Could you check a few things on this model? Use its own coordinates, in mm. A direction names the side the tool comes from. Give positions to 0.01 mm unless a question says otherwise; leave off trailing zeros. Loops run counter-clockwise (first coordinate to the right, second up) from the corner with the lowest first, then second, coordinate; pieces in that order, holes last. Notation, with made-up numbers: (25, 37) - (68, 37) arc R25 ccw to (68, 63) - close; hole circle Ø3 at (-20, -14). An arc over 180 degrees is marked (long way). Use CSV: the item, a comma, the result in double quotes.
from build123d import *

# Parameters (mm, degrees)
SKETCH1_W       = 10
SKETCH1_H       = 16.5
MAIN_BODY_DEPTH = 12.2
M_BASE_DEPTH    = 4.95
SKETCH12_W      = 4.5
SKETCH12_H      = 1
MO_CUT_1_DEPTH  = 6
SKETCH13_W      = 1
SKETCH13_H      = 1
MO_PINS_DEPTH   = 5


with BuildPart() as part:
    # Sketch1 → Main_Body (new body)
    with BuildSketch(Plane(origin=(0, 0, 0), x_dir=(1, 0, 0), z_dir=(0, 1, 0))):
        with Locations((0, 8.25)):
            Rectangle(SKETCH1_W, SKETCH1_H)
    extrude(amount=MAIN_BODY_DEPTH)

    # Sketch11 → M_Base (add, symmetric)
    with BuildSketch(Plane(origin=(0, 0, 0), x_dir=(0, 0, -1), z_dir=(1, 0, 0))):
        Polygon((0.7, 12.2), (1.063619422, 17.4), (22.553619422, 17.4), (22.553619422, 10.8), (16.5, 10.8), (16.5, 12.2), align=None)
    extrude(amount=M_BASE_DEPTH, both=True)

    # Sketch12 → MO_Cut_1 (cut)
    with BuildSketch(Plane(origin=(0, 0, -22.553619422), x_dir=(-1, 0, 0), z_dir=(0, 0, -1))):
        with Locations((0, 16.9)):
            Rectangle(SKETCH12_W, SKETCH12_H)
        Polygon((-3.45, 15.1), (3.45, 15.1), (3.45, 13.6), (2.9, 13.6), (2.9, 11.9), (-2.9, 11.9), (-2.9, 13.6), (-3.45, 13.6), align=None)
    extrude(amount=-MO_CUT_1_DEPTH, mode=Mode.SUBTRACT)

    # Sketch13 → MO_Pins (add)
    with BuildSketch(Plane(origin=(0, 0, -16.553619422), x_dir=(-1, 0, 0), z_dir=(0, 0, -1))):
        with Locations((-1.25, 13.8)):
            Rectangle(SKETCH13_W, SKETCH13_H)
        with Locations((1.25, 13.8)):
            Rectangle(SKETCH13_W, SKETCH13_H)
    extrude(amount=MO_PINS_DEPTH)


solid = part.part
1) Suppose I cut it at A-A (z = -18.5). Please give me the cut outline in (x, y), plus the area to 3 significant figures.
Answer below:
outline,"(-4.95, 10.8) - (4.95, 10.8) - (4.95, 17.4) - (2.25, 17.4) - (2.25, 16.4) - (-2.25, 16.4) - (-2.25, 17.4) - (-4.95, 17.4) - close; (-1.75, 13.3) - (-0.75, 13.3) - (-0.75, 14.3) - (-1.75, 14.3) - close; (0.75, 13.3) - (1.75, 13.3) - (1.75, 14.3) - (0.75, 14.3) - close; hole (-3.45, 13.6) - (-2.9, 13.6) - (-2.9, 11.9) - (2.9, 11.9) - (2.9, 13.6) - (3.45, 13.6) - (3.45, 15.1) - (-3.45, 15.1) - close"
area,"42.6 mm2"
2) Suppose I cut it at D-D (x = 4.25). Please give me the cut outline in (y, z), plus the area to 3 significant figures.
Answer below:
outline,"(0, -16.5) - (10.8, -16.5) - (10.8, -22.55) - (17.4, -22.55) - (17.4, -1.06) - (12.2, -0.7) - (12.2, 0) - (0, 0) - close"
area,"322 mm2"
3) Suppose I cut it at C-C (y = 3). Please give me the cut outline in (x, z).
Answer below:
outline,"(-5, -16.5) - (5, -16.5) - (5, 0) - (-5, 0) - close"
4) We'd pull the mould along X, two halves only. Please class faces 1 (the flat face through (-3.45, 14, -20)), 2 (the flat face through (0, 17.4, -12)), 3 (the flat face through (5, 6, -8)): +X half, -X half, draft (parallel to the pull), parting line (faces both ways), or undercut.
Answer below:
face 1,"undercut"
face 2,"draft"
face 3,"+X half"
5) Suppose I cut it at B-B (x = -0.5). Please give me the cut outline in (y, z).
Answer below:
outline,"(0, -16.5) - (10.8, -16.5) - (10.8, -22.55) - (11.9, -22.55) - (11.9, -16.55) - (15.1, -16.55) - (15.1, -22.55) - (16.4, -22.55) - (16.4, -16.55) - (17.4, -16.55) - (17.4, -1.06) - (12.2, -0.7) - (12.2, 0) - (0, 0) - close"
6) I need wall thicknesses on line 1 along Y through (x, z) = (-2.5, -21.5); line 2 along Z through (x, y) = (-3, 13); line 3 along Z through (x, y) = (2.5, 4.25). Which ranges of each line are inside material? Lowest first, please.
Answer below:
line 1,"y = 10.8 to 11.9, 15.1 to 17.4"
line 2,"z = -22.55 to -0.76"
line 3,"z = -16.5 to 0"
7) Which directions (+Z, -Z, +X, -X, +Y, -Y) give clear straight access to the entire face, cutting with the end or side of a thin tool? Please do faces 4 (the flat face through (0, 6, 0)), 5 (the flat face through (2.25, 17, -20)), 6 (the flat face through (2.9, 13, -20)).
Answer below:
face 4,"+Z, +X, -X, +Y, -Y"
face 5,"-Z, +Y"
face 6,"-Z"
8) I'm going to push flat-ended pins straight in: P1, Ø1, axis at y = 15.5, z = -17.5, coming from the +X side; P2, Ø0.8, axis at x = 1, y = 17, coming from the -Z side; P3, Ø0.5, axis at x = 1, z = -18.5, coming from the +Y side. Where does each tip first touch, or does it pass through?
Answer below:
P1,"stops at x = 4.95"
P2,"stops at z = -16.55"
P3,"stops at y = 16.4"
